Solid Edge part; units mm, degrees
sketch "Sketch1" plane through (0, 0, 0) normal (0, -1, 0) x (1, 0, 0)
  line L0 (53.5, 0) -> (0, 0)
  line L1 (0, 0) -> (0, 15)
  line L2 (0, 15) -> (53.5, 15)
  line L3 (53.5, 15) -> (53.5, 0)
extrude "Protrusion1" add sketch "Sketch1" along normal blind 5
sketch "Sketch2" plane through (18.75, 0, 7.5) normal (0, 1, 0) x (-1, 0, 0)
  line L0 (13.75, -7.5) -> (13.75, 7.5)
  line L1 (13.75, 7.5) -> (18.75, 7.5)
  line L2 (18.75, 7.5) -> (18.75, -7.5)
  line L3 (18.75, -7.5) -> (13.75, -7.5)
extrude "ExtrudedProtrusion_3" add sketch "Sketch2" along normal blind 15
sketch "Sketch3" plane through (0, 5, 7.5) normal (-1, 0, 0) x (0, -1, 0)
  circle A0 centre (-3, 0) radius 4
extrude "Cutout1" cut sketch "Sketch3" against normal through all
fillet "Round1" radius 7 2 edges at (2.5, 15, 15) (2.5, 15, 0)
mirror "Mirror1" about plane through (26.75, 5, 7.5) normal (-1, 0, 0) of "ExtrudedProtrusion_3", "Cutout1"
fillet "Round2" radius 7 2 edges at (51, 15, 15) (51, 15, 0)
Check sheet for the modelled part. Datum: model origin and axes. Units: mm. A direction names the side the tool comes from. Coordinates: 2 decimals unless noted, no trailing zeros. Loops run counter-clockwise (first coordinate to the right, second up) from the corner with the lowest first, then second, coordinate; pieces in that order, holes last. Notation, with made-up numbers: (47.5, 60) -> (96.5, 60) arc R20 cw to (96.5, 86) -> close; hole circle Ø2 at (-16.75, 39). An arc over 180 degrees is marked (long way). Write item = value, one per line. Start each with the question number.
1. Section check C-C on z = 2. Record the cut outline in (x, y), then the cut area to 3 significant figures.
2. Section check A-A on z = 7.5. Record the cut outline in (x, y), then the cut area to 4 significant figures.
3. Depth check by flat-ended pin: P1, Ø4.5, axis at x = 20, z = 4, coming from the +Y side; P2, Ø10, axis at x = 39, y = 11, coming from the +Z side. Enter the tip coordinate at first touch or a pass-through.
4. Draft check along X on faces 1 (the flat face through (27, 0, 7)), 2 (the flat face through (0, 3, 7)), 3 (the flat face through (2.5, 15, 7.5)). Enter one of: released by +X, released by -X, zero draft, split by the parting line, or undercut.
5. Section check D-D on z = 12. Record the cut outline in (x, y), then the cut area to 3 significant figures.
6. Section check B-B on x = 50. Record the cut outline in (y, z), then the cut area to 3 significant figures.
7. Tool access check on faces 4 (the flat face through (5, 4, 6)), 5 (the flat face through (51, 15, 7.5)). Record the directions out of +Z, -Z, +X, -X, +Y, -Y that give a thin tool (end or side, any length) a straight path to the whole face; none if there is none.
8. Material ranges on line 1 (X direction, y = 1.75, z = 8.5); line 2 (Z direction, x = 50.8, y = 8); line 3 (Y direction, x = 10, z = 2.5), recorded low to high.
Responses:
q1.outline = (0, -5) -> (53.5, -5) -> (53.5, 12.9) -> (48.5, 12.9) -> (48.5, 0) -> (5, 0) -> (5, 12.9) -> (0, 12.9) -> close
q1.area = 396 mm2
q2.outline = (0, -5) -> (53.5, -5) -> (53.5, 4) -> (48.5, 4) -> (48.5, 0) -> (5, 0) -> (5, 4) -> (0, 4) -> close; (0, 12) -> (5, 12) -> (5, 15) -> (0, 15) -> close; (48.5, 12) -> (53.5, 12) -> (53.5, 15) -> (48.5, 15) -> close
q2.area = 337.5 mm2
q3.P1 = 0
q3.P2 = through
q4.face_1 = undercut
q4.face_2 = released by -X
q4.face_3 = zero draft
q5.outline = (0, -5) -> (53.5, -5) -> (53.5, 13.74) -> (48.5, 13.74) -> (48.5, 0) -> (5, 0) -> (5, 13.74) -> (0, 13.74) -> close
q5.area = 405 mm2
q6.outline = (-5, 0) -> (8, 0) arc R7 ccw to (15, 7) -> (15, 8) arc R7 ccw to (8, 15) -> (-5, 15) -> close; hole circle Ø8 at (8, 7.5)
q6.area = 229 mm2
q7.face_4 = +Z, -Z, +Y
q7.face_5 = +Z, -Z, +X, -X, +Y
q8.line_1 = 0 to 5, 48.5 to 53.5
q8.line_2 = 0 to 3.5, 11.5 to 15
q8.line_3 = -5 to 0
